Source: CAD feature listing. Evaluate the final solid. Frame: model axes, mm. A direction names the side the tool comes from. Round coordinates to 2 decimals unless told otherwise and drop trailing zeros. Loops run counter-clockwise (first coordinate to the right, second up) from the corner with the lowest first, then second, coordinate; pieces in that order, holes last. Notation, with made-up numbers: M -29,14.25 L 22,14.25 A26 ccw 22,31.25 Z; hole C 85,76.5 d7. An arc over 180 degrees is marked long. Answer as a JSON object with one key per item and string values.
Autodesk Inventor part; units mm, degrees
ref_plane "YZ Plane" through (0, 0, 0) normal (1, 0, 0) x (0, 1, 0)
ref_plane "XZ Plane" through (0, 0, 0) normal (0, 1, 0) x (-1, 0, 0)
ref_plane "XY Plane" through (0, 0, 0) normal (0, 0, 1) x (1, 0, 0)
sketch "Sketch1" plane through (0, 0, 0) normal (0, 1, 0) x (-1, 0, 0)
  circle A0 centre (0, 0) radius 900
  circle A1 centre (0, 0) radius 1000
  dimension "d0" = 1800
  dimension "d1" = 100
extrude "Extrusion1" add sketch "Sketch1" along normal blind 20
sketch "Sketch2" plane through (0, 20, 0) normal (0, 1, 0) x (1, 0, 0)
  circle A0 centre (950, 0) radius 40
  circle A1 centre (-474.7961, 824.5017) radius 40
  circle A2 centre (-475.9164, -823.8556) radius 40
  line L0 (0, 0) -> (943.1963, 0) construction
  dimension "d7" = 360
  dimension "d11" = 950
  dimension "d13" = 80
  dimension "d14" = 80
extrude "Extrusion2" add sketch "Sketch2" along normal blind 20
sketch "Sketch3" plane through (0, 20, 0) normal (0, 1, 0) x (1, 0, 0)
  point P0 (0, 0)
Item 1: Contact query for flat-ended pins moving along their axis: pin 1 Ø5 at (y, z) = (7, -574.5) entering from -X; pin 2 Ø4 at (x, y) = (553, 9) entering from -Z; pin 3 Ø8 at (x, y) = (341.5, 13.5) entering from +Z. Output: stop coordinate, or through.
Answer sheet:
{"pin 1": "stops at x = -820.25", "pin 2": "stops at z = -834.51", "pin 3": "stops at z = 941.33"}
Item 2: Section C-C on x = 950. Return the cut outline in (y, z), then the cut area to 3 significant figures.
Answer sheet:
{"outline": "M 0,-312.25 L 20,-312.25 L 20,-40 L 40,-40 L 40,40 L 20,40 L 20,312.25 L 0,312.25 Z", "area": "14,100 mm²"}
Item 3: Line query: probe 1 along Z at (x, y) = (0, 7); probe 2 along Z at (x, y) = (156.5, 5.5); probe 3 along X at (y, z) = (4, -61). Output: solid intervals per line, ascending. Write a range as from..to.
Answer sheet:
{"probe 1": "z = -1000..-900, 900..1000", "probe 2": "z = -987.68..-886.29, 886.29..987.68", "probe 3": "x = -998.14..-897.93, 897.93..998.14"}
Item 4: Section B-B on z = -172. Return the cut outline in (x, y).
Answer sheet:
{"outline": "M -985.1,0 L -883.41,0 L -883.41,20 L -985.1,20 Z; M 883.41,0 L 985.1,0 L 985.1,20 L 883.41,20 Z"}
Item 5: Section A-A on x = 0. Return the cut outline in (y, z).
Answer sheet:
{"outline": "M 0,-1000 L 20,-1000 L 20,-900 L 0,-900 Z; M 0,900 L 20,900 L 20,1000 L 0,1000 Z"}
Item 6: Pull-direction query (Z, two-part tool) for faces 1 (the cylindrical face through (899.13, 9.86, -39.57)), 2 (the cylindrical face through (-483.47, 29.86, -863.55)), 3 (the flat face through (-475, 40, -825)), 4 (the cylindrical face through (986.95, 29.86, -15.32)); classes: pulls with the +Z half, pulls with the -Z half, needs draft (parallel to the pull), parting line crosses it, or undercut.
Answer sheet:
{"face 1": "undercut", "face 2": "undercut", "face 3": "needs draft", "face 4": "parting line crosses it"}
Item 7: Access query for faces 5 (the cylindrical face through (-505.4, 29.86, 850.89)), 6 (the flat face through (-476, 40, 823)). Directions: +Z, -Z, +X, -X, +Y, -Y. A direction counts if a zero-diameter tool reaches every point of the face in a straight line with its end or side. Return the directions, or none.
Answer sheet:
{"face 5": "+Y", "face 6": "+Z, -Z, +X, -X, +Y"}
